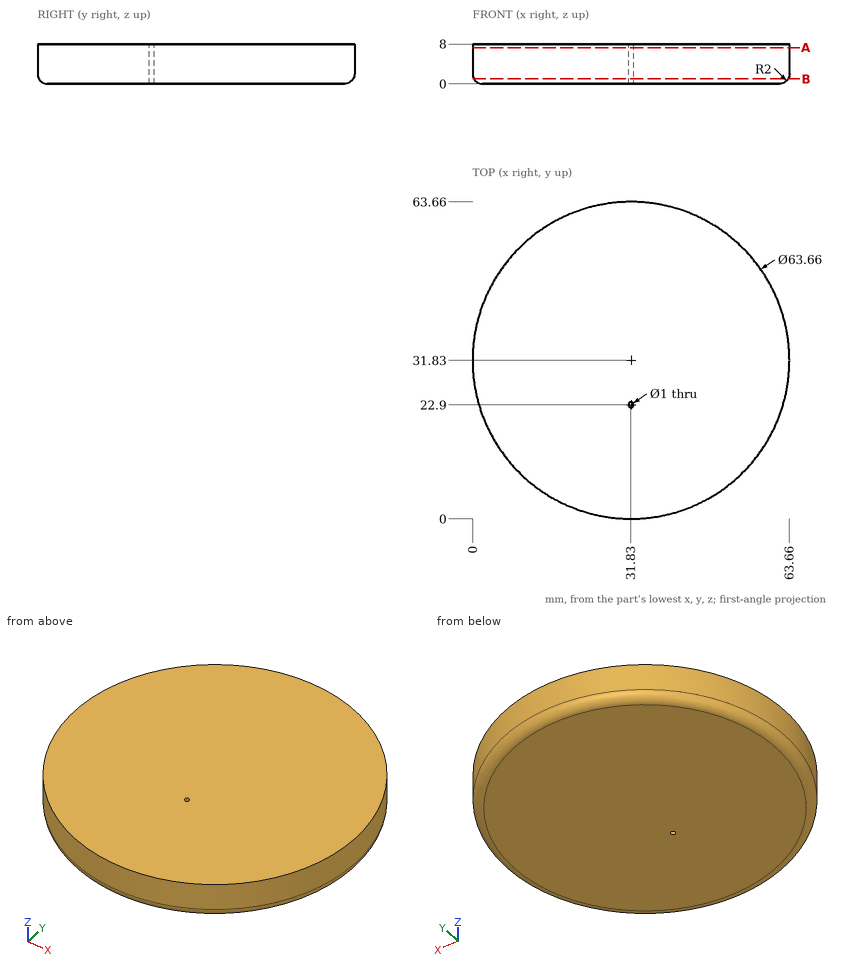
The figure shows three views and two pictorial views of one solid part (mm, origin at its lowest corner). Answer the questions. Give positions to 0.01 mm unless a question says otherwise; leave off trailing zeros. Write each loop counter-clockwise with the first axis right and the second up, starting at its lowest first coordinate (ties: lowest second). Pieces come first, ordered by that corner, then holes. Notation, with made-up numbers: M 72.25,85 L 91.25,85 A23 cw 91.25,93 Z; hole C 75,64 d4. An arc over 180 degrees is marked long. One line per item, written item: value. Start each with the question number.
(1) Flat-ended cylindrical pins translate along their axes: pin 1 Ø3 at (y, z) = (51, 2.5) entering from -X; pin 2 Ø4 at (x, z) = (9, 6.5) entering from -Y; pin 3 Ø2 at (x, z) = (12, 2.5) entering from +Y. Find the tip coordinate at first contact, or state that the pin passes through.
(2) Find section B-B (z = 1). Determine the outline of the cut face in (x, y), plus the area to 3 significant figures.
(3) Find the intervals of material crossed by line 1 (Y direction, x = 31.83, z = 5.5); line 2 (Y direction, x = 44, z = 2.75); line 3 (X direction, y = 4, z = 2), in increasing order.
(4) Find section A-A (z = 7.25). Determine the outline of the cut face in (x, y), plus the area to 3 significant figures.
Results below:
1. pin 1: stops at x = 5.36
1. pin 2: stops at y = 7.76
1. pin 3: stops at y = 57.49
2. outline: C 31.83,31.83 d63.12; hole C 31.83,22.9 d1
2. area: 3,130 mm^2
3. line 1: y = 0 to 22.4, 23.4 to 63.66
3. line 2: y = 2.42 to 61.24
3. line 3: x = 16.38 to 47.28
4. outline: C 31.83,31.83 d63.66; hole C 31.83,22.9 d1
4. area: 3,180 mm^2
